Design review of the part built by this model. Coordinates are the model's own, in mm. Face numbers are marked on the shaded views. A direction names the side the tool comes from. Give positions to 0.01 mm unless a question says otherwise; leave off trailing zeros. Write each loop counter-clockwise with the first axis right and the second up, starting at its lowest first coordinate (ties: lowest second). Pieces come first, ordered by that corner, then holes. Notation, with made-up numbers: M 79,60.25 L 135,60.25 A29 ccw 135,92.25 Z; hole C 68,60 d3. An arc over 180 degrees is marked long. One line per item, written item: value. Start each with the question number.
```python
from build123d import *

# Parameters (mm, degrees)
F0_R     = 26.5
F1_DEPTH = 20
F2_R     = 12.44
F3_DEPTH = 5.2
F4_R     = 10
F5_DEPTH = 7.6
F6_R     = 12.44
F7_DEPTH = 4.9
F8_R     = 0.5
F9_R     = 0.2


with BuildPart() as f1:
    # F0 (on Top) → F1 (new body)
    with BuildSketch(Plane.XY):
        Circle(F0_R)
    extrude(amount=F1_DEPTH)

    # F2 (on face) → F3 (join)
    with BuildSketch(Plane.XY.offset(20)):
        Circle(F2_R)
    extrude(amount=F3_DEPTH)

    # F4 (on face) → F5 (join)
    with BuildSketch(Plane.XY.offset(25.2)):
        Circle(F4_R)
    extrude(amount=F5_DEPTH)

    # F6 (on face) → F7 (join)
    with BuildSketch(Plane.XY.offset(32.8)):
        Circle(F6_R)
    extrude(amount=F7_DEPTH)

    # F8
    f8_edges = [f1.edges().sort_by_distance(p)[0] for p in [
        (-12.44, 0, 37.7),
        (-26.5, 0, 20),
        (-26.5, 0, 0),
    ]]
    fillet(f8_edges, radius=F8_R)

    # F9
    f9_edges = [f1.edges().sort_by_distance(p)[0] for p in [
        (-12.44, 0, 25.2),
        (-12.44, 0, 32.8),
    ]]
    fillet(f9_edges, radius=F9_R)


solid = f1.part
```
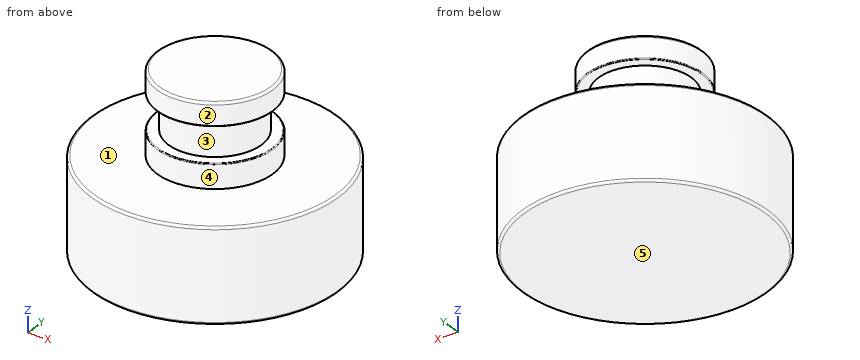
Q1. The part is to be moulded in two halves that separate along Y. For the marked faces 1 and 2, say which applies: pulls with the +Y half, pulls with the -Y half, needs draft (parallel to the pull), parting line crosses it, or undercut.
Q2. For P1, Ø1.5, axis at x = -17.5, y = 6.5, coming from the +Z side; P2, Ø12, axis at x = 1, y = -4.5, coming from the -Z side; P3, Ø10, axis at y = 18, z = 4.5, coming from the +X side; P4, Ø8, axis at y = -21, z = 21, coming from the -X side, all flat-tipped, find the tip position at first contact; note any pin that passes through.
Q3. Machinability: for the marked faces 3, 4 and 5, which of the approach directions +Z, -Z, +X, -X, +Y, -Y give a long, thin tool a straight path to every point of the face, cutting with its end or side? Answer none if there is none.
Q4. Take a section at A-A, the plane y = 0. Give the boundary of the cut face in (x, z).
Q5. Take a section at D-D, the plane z = 18.5. Give the boundary of the cut face in (x, y).
Q6. Wall thickness on line 1 (Z direction, x = -9.5, y = -15); line 2 (X direction, y = 23.5, z = 10.5): over which ranges is each line inside the solid? List them lowest first. Write a range as from..to.
Q7. Take a section at C-C, the plane z = 27.5. Give the boundary of the cut face in (x, y).
Results list:
1. face 1: needs draft
1. face 2: parting line crosses it
2. P1: stops at z = 20
2. P2: stops at z = 0
2. P3: stops at x = 23.09
2. P4: stops at x = -20.1
3. face 3: none
3. face 4: +Z
3. face 5: -Z, +X, -X, +Y, -Y
4. outline: M -26.5,0.5 A0.5 ccw -26,0 L 26,0 A0.5 ccw 26.5,0.5 L 26.5,19.5 A0.5 ccw 26,20 L 12.44,20 L 12.44,25 A0.2 ccw 12.24,25.2 L 10,25.2 L 10,32.8 L 12.24,32.8 A0.2 ccw 12.44,33 L 12.44,37.2 A0.5 ccw 11.94,37.7 L -11.94,37.7 A0.5 ccw -12.44,37.2 L -12.44,33 A0.2 ccw -12.24,32.8 L -10,32.8 L -10,25.2 L -12.24,25.2 A0.2 ccw -12.44,25 L -12.44,20 L -26,20 A0.5 ccw -26.5,19.5 Z
5. outline: C 0,0 d53
6. line 1: z = 0..20
6. line 2: x = -12.25..12.25
7. outline: C 0,0 d20
